```python
from build123d import *

# Parameters (mm, degrees)
SKETCH_1_W      = 38
SKETCH_1_H      = 16
EXTRUDE_1_DEPTH = 5
SKETCH_2_W      = 14
SKETCH_2_H      = 5
EXTRUDE_2_DEPTH = 25
SKETCH_3_W      = 14
SKETCH_3_H      = 30
EXTRUDE_3_DEPTH = 8


with BuildPart() as part:
    # 草图1 → 凸台-拉伸1 (new body)
    with BuildSketch(Plane.XY):
        Rectangle(SKETCH_1_W, SKETCH_1_H)
    extrude(amount=EXTRUDE_1_DEPTH)

    # 草图2 → 凸台-拉伸2 (add)
    with BuildSketch(Plane.XY.offset(5)):
        Rectangle(SKETCH_2_W, SKETCH_2_H)
    extrude(amount=EXTRUDE_2_DEPTH)

    # 草图3 → 凸台-拉伸3 (add)
    with BuildSketch(Plane.XY.offset(30)):
        Rectangle(SKETCH_3_W, SKETCH_3_H)
    extrude(amount=EXTRUDE_3_DEPTH)


solid = part.part
```
Check sheet for the modelled part. Datum: model origin and axes. Units: mm. A direction names the side the tool comes from. Round coordinates to 2 decimals unless told otherwise and drop trailing zeros. Loops run counter-clockwise (first coordinate to the right, second up) from the corner with the lowest first, then second, coordinate; pieces in that order, holes last. Notation, with made-up numbers: (-18.5, 42) - (31.5, 42) arc R19 ccw to (31.5, 53) - close; hole circle Ø11 at (7, 44). An arc over 180 degrees is marked (long way). Answer as a JSON object with one key per item and string values. Group by question number.
Q1. Sectioned sample at B-B, the plane y = -0.75. Enter the section's corners in (x, z).
Q2. Sectioned sample at A-A, the plane y = 6. Enter the section's corners in (x, z).
Q3. Gauge pin test, flat ends, axial feed: P1, Ø3, axis at y = 10, z = 5, coming from the +X side; P2, Ø5, axis at y = -5, z = 31.5, coming from the -X side; P3, Ø4, axis at x = -5, z = 1.5, coming from the -Y side; P4, Ø11, axis at x = 1.5, z = 19, coming from the +Y side. Record the tip position at first contact, or that the pin passes through.
Q4. Scan lines: line 1 along Z through (x, y) = (0, -6.25); line 2 along Z through (x, y) = (-16, -4); line 3 along X through (y, z) = (3.75, 35). Record each from-to range of solid material in increasing order. Write a range as [from, to].
Q5. Mould release check, pull along Z, two halves, no side actions. Record for faces 5 (the face through (0, -15, 34)), 6 (the face through (0, 0, 0)), 7 (the face through (0, 2.5, 17)): released by +Z, released by -Z, zero draft, split by the parting line, or undercut.
Q6. Set-up check for faces 1 (the face through (0, 4, 5)), 2 (the face through (0, 8, 2)), 3 (the face through (-7, 0, 28)), 4 (the face through (0, -8, 2)): record each of +Z, -Z, +X, -X, +Y, -Y from which the full face is reachable in a straight line by a thin tool's end or side.
Q7. Sectioned sample at C-C, the plane x = 5.5. Enter the section's corners in (y, z).
Q8. Sectioned sample at D-D, the plane z = 35.5. Enter the section's corners in (x, y), plus the area to 3 significant figures.
Solution:
{
 "1": {"outline": "(-19, 0) - (19, 0) - (19, 5) - (7, 5) - (7, 38) - (-7, 38) - (-7, 5) - (-19, 5) - close"},
 "2": {"outline": "(-19, 0) - (19, 0) - (19, 5) - (-19, 5) - close; (-7, 30) - (7, 30) - (7, 38) - (-7, 38) - close"},
 "3": {"P1": "passes through", "P2": "stops at x = -7", "P3": "stops at y = -8", "P4": "stops at y = 2.5"},
 "4": {"line 1": "z = [0, 5], [30, 38]", "line 2": "z = [0, 5]", "line 3": "x = [-7, 7]"},
 "5": {"face 5": "zero draft", "face 6": "released by -Z", "face 7": "undercut"},
 "6": {"face 1": "none", "face 2": "-Z, +X, -X, +Y", "face 3": "+Z, -X, +Y, -Y", "face 4": "-Z, +X, -X, -Y"},
 "7": {"outline": "(-15, 30) - (-2.5, 30) - (-2.5, 5) - (-8, 5) - (-8, 0) - (8, 0) - (8, 5) - (2.5, 5) - (2.5, 30) - (15, 30) - (15, 38) - (-15, 38) - close"},
 "8": {"outline": "(-7, -15) - (7, -15) - (7, 15) - (-7, 15) - close", "area": "420 mm²"}
}
